```python
from build123d import *

# Parameters (mm, degrees)
SKETCH_1_R          = 31.5
SKETCH_1_R_2        = 29
EXTRUDE_1_DEPTH     = 14
EXTRUDE_START       = -14
EXTRUDE_2_DEPTH     = 14
SKETCH_3_R          = 1.5
CUT_EXTRUDE_1_DEPTH = 50.124840967
FILLET_1_R          = 3


with BuildPart() as part:
    # 草图1 → 凸台-拉伸1 (new body)
    with BuildSketch(Plane.XY):
        Circle(SKETCH_1_R)
        Circle(SKETCH_1_R_2, mode=Mode.SUBTRACT)
    extrude(amount=EXTRUDE_1_DEPTH)

    # 草图2 → 凸台-拉伸2 (add)
    with BuildSketch(Plane.XY.offset(14).offset(EXTRUDE_START)):
        with BuildLine():
            ThreePointArc((-28.627224802, 13.142754664), (-27.279800219, 15.75), (-25.695571815, 18.220526586))
            ThreePointArc((-25.695571815, 18.220526586), (-30.310889132, 17.5), (-28.627224802, 13.142754664))
        make_face()
        with BuildLine():
            ThreePointArc((-2.931652987, 31.36328125), (0, 31.5), (2.931652987, 31.36328125))
            ThreePointArc((2.931652987, 31.36328125), (0, 35), (-2.931652987, 31.36328125))
        make_face()
        with BuildLine():
            ThreePointArc((28.627224802, 13.142754664), (30.310889132, 17.5), (25.695571815, 18.220526586))
            ThreePointArc((25.695571815, 18.220526586), (27.279800219, 15.75), (28.627224802, 13.142754664))
        make_face()
        with BuildLine():
            ThreePointArc((25.695571815, -18.220526586), (30.310889132, -17.5), (28.627224802, -13.142754664))
            ThreePointArc((28.627224802, -13.142754664), (27.279800219, -15.75), (25.695571815, -18.220526586))
        make_face()
        with BuildLine():
            ThreePointArc((2.931652987, -31.36328125), (0, -31.5), (-2.931652987, -31.36328125))
            ThreePointArc((-2.931652987, -31.36328125), (0, -35), (2.931652987, -31.36328125))
        make_face()
        with BuildLine():
            ThreePointArc((-25.695571815, -18.220526586), (-27.279800219, -15.75), (-28.627224802, -13.142754664))
            ThreePointArc((-28.627224802, -13.142754664), (-30.310889132, -17.5), (-25.695571815, -18.220526586))
        make_face()
    extrude(amount=EXTRUDE_2_DEPTH)

    # 草图3 → 切除-拉伸1 (cut, through all)
    with BuildSketch(Plane.XY.offset(14)):
        with Locations((0, 32)):
            Circle(SKETCH_3_R)
        with Locations((-27.712812921, 16)):
            Circle(SKETCH_3_R)
        with Locations((-27.712812921, -16)):
            Circle(SKETCH_3_R)
        with Locations((0, -32)):
            Circle(SKETCH_3_R)
        with Locations((27.712812921, -16)):
            Circle(SKETCH_3_R)
        with Locations((27.712812921, 16)):
            Circle(SKETCH_3_R)
    extrude(amount=-CUT_EXTRUDE_1_DEPTH, mode=Mode.SUBTRACT)

    # 圆角1
    fillet_1_edges = [part.edges().sort_by_distance(p)[0] for p in [
        (-25.695571815, 18.220526586, 7),
        (-28.627224802, 13.142754664, 7),
        (2.931652987, 31.36328125, 7),
        (-2.931652987, 31.36328125, 7),
        (28.627224802, 13.142754664, 7),
        (25.695571815, 18.220526586, 7),
        (25.695571815, -18.220526586, 7),
        (28.627224802, -13.142754664, 7),
        (-2.931652987, -31.36328125, 7),
        (2.931652987, -31.36328125, 7),
        (-28.627224802, -13.142754664, 7),
        (-25.695571815, -18.220526586, 7),
    ]]
    fillet(fillet_1_edges, radius=FILLET_1_R)


solid = part.part
```
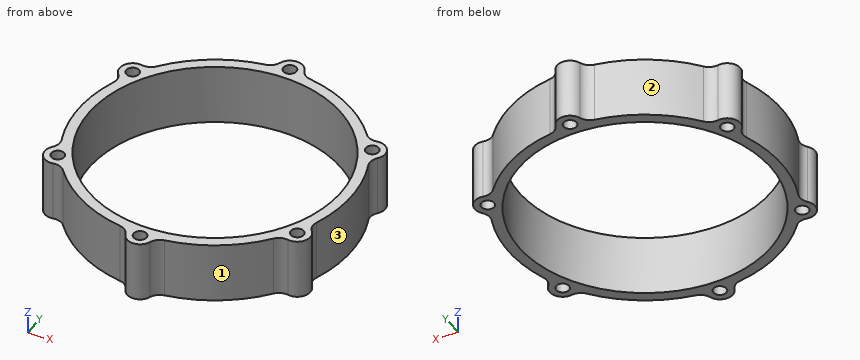
Model file for the job. Use its own axes, mm. Face numbers are marked on the shaded views. Coordinates: 2 decimals unless noted, no trailing zeros. Write each loop counter-clockwise with the first axis right and the second up, starting at its lowest first coordinate (ties: lowest second). Pieces come first, ordered by that corner, then holes. Notation, with made-up numbers: (3.5, 42.5) - (50.5, 42.5) arc R24 cw to (50.5, 65.5) - close; hole circle Ø1 at (-16, 74). An arc over 180 degrees is marked (long way). One line per question, with ' | ' between items. Start each with the question number.
Q1. Cut at A-A, the plane x = 0. List the corners of the cut face in (y, z), then the cut area to 3 significant figures.
Q2. Cut at D-D, the plane y = 16. List the corners of the cut face in (x, z), then the cut area to 3 significant figures.
Q3. Drill centre lines: line 1 (X direction, y = -25, z = 11); line 2 (X direction, y = -11, z = 3); line 3 (Y direction, x = -2, z = 2.5). Where is each one in solid material? Low to high. Write a range as [from, to].
Q4. Pin check, flat tips, straight feed: pin 1 (1 mm diameter, centred on x = -1, z = 6.5, fed in from -Y); pin 2 (2 mm diameter, centred on y = -9, z = 2, fed in from +X). Stop position of each tip, or through.
Q5. Cut at B-B, the plane y = 0. List the corners of the cut face in (x, z), then the cut area to 3 significant figures.
Q6. Cut at C-C, the plane x = 20. List the corners of the cut face in (y, z), then the cut area to 3 significant figures.
Q7. Pull direction Y, two halves, no side cores. Call the marked faces 1, 2 and 3: pulls with the +Y half, pulls with the -Y half, needs draft (parallel to the pull), parting line crosses it, or undercut.
Answer below:
1) outline: (-35, 0) - (-33.5, 0) - (-33.5, 14) - (-35, 14) - close; (-30.5, 0) - (-29, 0) - (-29, 14) - (-30.5, 14) - close; (29, 0) - (30.5, 0) - (30.5, 14) - (29, 14) - close; (33.5, 0) - (35, 0) - (35, 14) - (33.5, 14) - close | area: 84.0 mm^2
2) outline: (-30.71, 0) - (-29.21, 0) - (-29.21, 14) - (-30.71, 14) - close; (-26.21, 0) - (-24.19, 0) - (-24.19, 14) - (-26.21, 14) - close; (24.19, 0) - (26.21, 0) - (26.21, 14) - (24.19, 14) - close; (29.21, 0) - (30.71, 0) - (30.71, 14) - (29.21, 14) - close | area: 98.7 mm^2
3) line 1: [-19.16, -14.7], [14.7, 19.16] | line 2: [-29.52, -26.83], [26.83, 29.52] | line 3: [-34.24, -28.93], [28.93, 34.24]
4) pin 1: y = -34.96 | pin 2: x = 30.47
5) outline: (-31.5, 0) - (-29, 0) - (-29, 14) - (-31.5, 14) - close; (29, 0) - (31.5, 0) - (31.5, 14) - (29, 14) - close | area: 70.0 mm^2
6) outline: (-24.34, 0) - (-21, 0) - (-21, 14) - (-24.34, 14) - close; (21, 0) - (24.34, 0) - (24.34, 14) - (21, 14) - close | area: 93.4 mm^2
7) face 1: pulls with the -Y half | face 2: pulls with the +Y half | face 3: undercut
